Could you check a few things on this drawing? It's one solid part, dimensions in mm from its lowest x, y, z. Coordinates: 2 decimals unless noted, no trailing zeros. Order: outer loops, then holes, each group sorted by start corner. A loop starts at its lowest first (then second) coordinate and runs counter-clockwise, first axis right, second up. Notation, with made-up numbers: M 3,26.25 L 20,26.25 A14 ccw 20,38.25 Z; hole C -24,7.25 d10. An arc over 180 degrees is marked long. One line per question, with ' | ' between items. Start each with the question number.
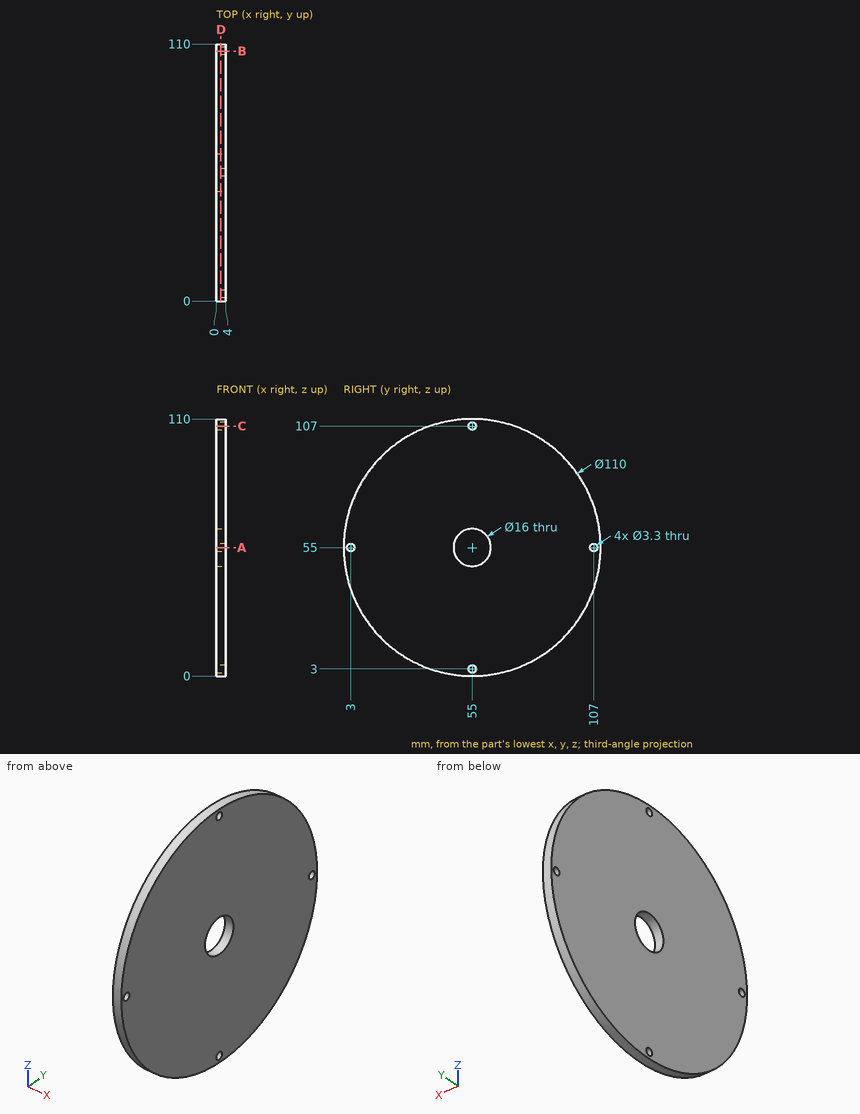
1. Imagine slicing it at D-D (x = 1.95). List the corners of the cut face in (y, z) for me.
2. Imagine slicing it at A-A (z = 55). List the corners of the cut face in (x, y) for me, then the cut area to 3 significant figures.
3. Imagine slicing it at B-B (y = 107). List the corners of the cut face in (x, z) for me, then the cut area to 3 significant figures.
4. I need wall thicknesses on line 1 (Y direction, x = 3, z = 55); line 2 (Z direction, x = 3.55, y = 15.5); line 3 (Z direction, x = 2.75, y = 90.5). Which ranges of each line are inside material? Lowest first, please.
5. Will these pins go through, and if not, where does the flat tip stop? pin 1 (3 mm diameter, centred on y = 3, z = 55, fed in from -X); pin 2 (8 mm diameter, centred on y = 26, z = 76, fed in from -X); pin 3 (1 mm diameter, centred on x = 1.5, z = 71, fed in from +Y); pin 4 (1 mm diameter, centred on x = 2.5, y = 57.5, fed in from -Z).
Entries:
1) outline: C 55,55 d110; hole C 3,55 d3.3; hole C 55,55 d16; hole C 55,3 d3.3; hole C 55,107 d3.3; hole C 107,55 d3.3
2) outline: M 0,0 L 4,0 L 4,1.35 L 0,1.35 Z; M 0,4.65 L 4,4.65 L 4,47 L 0,47 Z; M 0,63 L 4,63 L 4,105.35 L 0,105.35 Z; M 0,108.65 L 4,108.65 L 4,110 L 0,110 Z | area: 350 mm²
3) outline: M 0,37.08 L 4,37.08 L 4,53.35 L 0,53.35 Z; M 0,56.65 L 4,56.65 L 4,72.92 L 0,72.92 Z | area: 130 mm²
4) line 1: 0 to 1.35, 4.65 to 47, 63 to 105.35, 108.65 to 110 | line 2: 16.73 to 93.27 | line 3: 12.99 to 97.01
5) pin 1: through | pin 2: x = 0 | pin 3: y = 107.77 | pin 4: z = 0.04
